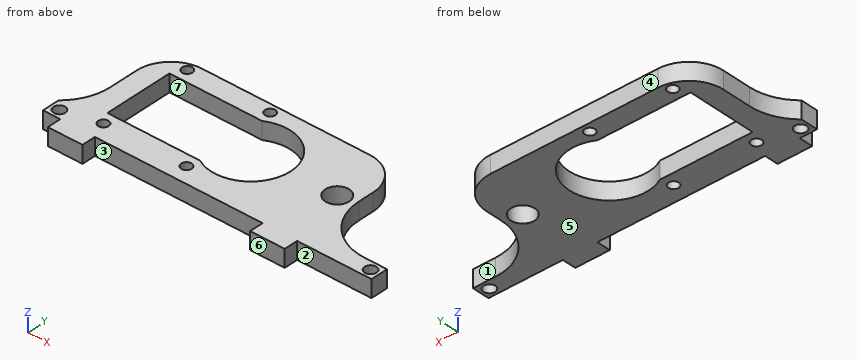
```python
from build123d import *

# Parameters (mm, degrees)
SKETCH1_R          = 3.45
SKETCH1_R_2        = 1.5
SKETCH1_R_3        = 1.7
BASE_FLANGE1_DEPTH = 5
FILLET1_R          = 15
FILLET2_R          = 15


# Sheet-metal steps are written as plain solids
with BuildPart() as part:
    # Sketch1 → Base-Flange1 (new body)
    with BuildSketch(Plane.XY):
        with BuildLine():
            Line((-28.5, 16), (20, 16))
            ThreePointArc((20, 16), (27.071067812, 13.071067812), (30, 6))
            Line((30, 6), (30, -13.5))
            Line((30, -13.5), (51.5, -13.5))
            Line((51.5, -13.5), (51.5, -18.5))
            Line((51.5, -18.5), (30, -18.5))
            Line((30, -18.5), (30, -22.5))
            Line((30, -22.5), (20, -22.5))
            Line((20, -22.5), (20, -18.5))
            Line((20, -18.5), (-28.5, -18.5))
            Line((-28.5, -18.5), (-28.5, -22.5))
            Line((-28.5, -22.5), (-38.5, -22.5))
            Line((-38.5, -22.5), (-38.5, -18.5))
            Line((-38.5, -18.5), (-43.5, -18.5))
            Line((-43.5, -18.5), (-43.5, -13.5))
            Line((-43.5, -13.5), (-38.5, -13.5))
            Line((-38.5, -13.5), (-38.5, 6))
            ThreePointArc((-38.5, 6), (-35.571067812, 13.071067812), (-28.5, 16))
        make_face()
        with Locations((25, 0)):
            Circle(SKETCH1_R, mode=Mode.SUBTRACT)
        with Locations((-6.5, 13.5)):
            Circle(SKETCH1_R_2, mode=Mode.SUBTRACT)
        with Locations((-30.5, 13.5)):
            Circle(SKETCH1_R_2, mode=Mode.SUBTRACT)
        with Locations((-30.5, -13.5)):
            Circle(SKETCH1_R_2, mode=Mode.SUBTRACT)
        with Locations((-6.5, -13.5)):
            Circle(SKETCH1_R_2, mode=Mode.SUBTRACT)
        with Locations((-41, -16)):
            Circle(SKETCH1_R_3, mode=Mode.SUBTRACT)
        with Locations((49, -16)):
            Circle(SKETCH1_R_3, mode=Mode.SUBTRACT)
        with BuildLine():
            Line((-5.678908346, 10), (-32.5, 10))
            Line((-32.5, 10), (-32.5, -10))
            Line((-32.5, -10), (-5.678908346, -10))
            ThreePointArc((-5.678908346, -10), (11.5, 0), (-5.678908346, 10))
        make_face(mode=Mode.SUBTRACT)
    extrude(amount=-BASE_FLANGE1_DEPTH)

    # Fillet1
    fillet1_edges = [part.edges().sort_by_distance(p)[0] for p in [
        (30, -13.5, -2.5),
    ]]
    fillet(fillet1_edges, radius=FILLET1_R)

    # Fillet2
    # the kernel refuses this fillet: 15 mm, written as the material it adds along each edge
    with BuildSketch(Plane(origin=(-38.5, -13.5, 0), x_dir=(0, 1, 0), z_dir=(0, 0, -1))) as fillet2_piece_1:
        with BuildLine():
            CenterArc((11.180339887, -15), FILLET2_R, 90, 48.189685104)
            Line((0, -5), (-0.223606798, -4.8))
            ThreePointArc((-0.223606798, -4.8), (-0.3, -2.5), (-0.3, 0))
            Line((-0.3, 0), (0, 0.3))
            Line((0, 0.3), (11.180339887, 0.3))
            Line((11.180339887, 0.3), (11.180339887, 0))
        make_face()
    extrude(amount=5)


solid = part.part
```
Build history of the part. All positions in model axes, mm. Face numbers are marked on the shaded views. A direction names the side the tool comes from. Round coordinates to 2 decimals unless told otherwise and drop trailing zeros. Order: outer loops, then holes, each group sorted by start corner. A loop starts at its lowest first (then second) coordinate and runs counter-clockwise, first axis right, second up. Notation, with made-up numbers: (17, 64) -> (39, 64) arc R18 cw to (39, 75) -> close; hole circle Ø7 at (67, 29). An arc over 180 degrees is marked (long way). Answer in a Markdown table with one row per item.
1) Band-saw the part on D-D on z = -3.5. Give the number of separate pieces and of enclosed holes in the cut face, and give its area (3 significant figures).
Values:
| item | result |
|---|---|
| separate pieces | 1 |
| enclosed holes | 8 |
| area | 1,650 mm2 |
2) Band-saw the part on A-A on x = 49. Give the cut face in (y, z), and give its area (3 significant figures).
Values:
| item | result |
|---|---|
| outline | (-18.5, -5) -> (-17.7, -5) -> (-17.7, 0) -> (-18.5, 0) -> close; (-14.3, -5) -> (-13.5, -5) -> (-13.5, 0) -> (-14.3, 0) -> close |
| area | 8.00 mm2 |
3) Which spindle directions (+Z, -Z, +X, -X, +Y, -Y) get a long thin tool onto all of the face, cutting with end or side? Do the marked faces 1, 2 and 3. Say none if no direction does.
Values:
| item | result |
|---|---|
| face 1 | +Z, -Z, +X, +Y |
| face 2 | +Z, -Z, +X, -Y |
| face 3 | +Z, -Z, -Y |
4) Pin check, flat tips, straight feed: P1, Ø2, axis at x = 49, y = -16, coming from the -Z side; P2, Ø1, axis at y = -8, z = -2, coming from the +X side; P3, Ø1.5, axis at x = 49.5, z = -2.5, coming from the +Y side; P4, Ø1.5, axis at y = -5, z = -2, coming from the -X side. Stop position of each tip, or through.
Values:
| item | result |
|---|---|
| P1 | through |
| P2 | x = 33.82 |
| P3 | y = -13.5 |
| P4 | x = -38.9 |
5) Band-saw the part on C-C on x = -6.5. Give the cut face in (y, z), and give its area (3 significant figures).
Values:
| item | result |
|---|---|
| outline | (-18.5, -5) -> (-15, -5) -> (-15, 0) -> (-18.5, 0) -> close; (-12, -5) -> (-10, -5) -> (-10, 0) -> (-12, 0) -> close; (10, -5) -> (12, -5) -> (12, 0) -> (10, 0) -> close; (15, -5) -> (16, -5) -> (16, 0) -> (15, 0) -> close |
| area | 42.5 mm2 |
6) Wall check: L1, parallel to Y at x = -6.5, z = -3.6; L2, parallel to Y at x = 0, z = -1.7; L3, parallel to X at y = 3, z = -3.25. Give the ranges that are in metal, low to high.
Values:
| item | result |
|---|---|
| L1 | -18.5 to -15, -12 to -10, 10 to 12, 15 to 16 |
| L2 | -18.5 to -11.5, 11.5 to 16 |
| L3 | -38.5 to -32.5, 11.1 to 23.3, 26.7 to 30 |
7) Mould opens along Y. For the marked faces 4, 5, 6 and 7 say: released by +Y, released by -Y, zero draft, split by the parting line, or undercut.
Values:
| item | result |
|---|---|
| face 4 | released by +Y |
| face 5 | zero draft |
| face 6 | released by -Y |
| face 7 | undercut |
8) Band-saw the part on B-B on y = -7. Give the cut face in (x, z).
Values:
| item | result |
|---|---|
| outline | (-39.25, -5) -> (-32.5, -5) -> (-32.5, 0) -> (-39.25, 0) -> close; (9.12, -5) -> (32.64, -5) -> (32.64, 0) -> (9.12, 0) -> close |
